Part model, mm, in its own coordinate system. A direction names the side the tool comes from. Give positions to 0.01 mm unless a question says otherwise; leave off trailing zeros. Order: outer loops, then holes, each group sorted by start corner. A loop starts at its lowest first (then second) coordinate and runs counter-clockwise, first axis right, second up. Notation, with made-up numbers: (83.25, -40) -> (95.25, -40) arc R11 cw to (95.25, -24) -> close; hole circle Ø9 at (68, 11.5). An arc over 180 degrees is marked (long way). Write item = value, one per line. Start each with the question number.
Item 1: Flat gauge pins, fed straight in: P1, Ø1.5, axis at x = 5, y = 18.5, coming from the +Z side; P2, Ø1.5, axis at y = 24, z = 7, coming from the -X side; P3, Ø0.6, axis at y = 28.5, z = 6.5, coming from the +X side; P4, Ø2.5, axis at x = 7.5, y = 5, coming from the +Z side. Where does each tip first touch, or does it go through?
Item 2: Band-saw the part on D-D on z = 1.5. Write the cut outline in (x, y).
Item 3: Tool access for faces 1 (the face through (8, 20, 6)), 2 (the face through (8, 28, 7)), 3 (the face through (5, 29, 6)): list every direction of +Z, -Z, +X, -X, +Y, -Y with a clear straight run to the whole face (end or side of a thin tool).
Item 4: Band-saw the part on B-B on x = 7.5. Write the cut outline in (y, z).
Item 5: Drill centre lines: line 1 along Y through (x, z) = (7.5, 3.2); line 2 along Y through (x, z) = (8.75, 5.5); line 3 along X through (y, z) = (15, 3.05). Where is each one in solid material? Low to high.
Item 6: Pull direction Y, two halves, no side cores. Call faces 4 (the face through (7, 0, 2)), 5 (the face through (9, 5, 2)), 6 (the face through (7, 29, 8)): +Y half, -Y half, draft (parallel to the pull), parting line (faces both ways), or undercut.
Item 7: Band-saw the part on C-C on z = 7. Write the cut outline in (x, y).
Item 8: Band-saw the part on A-A on y = 5. Write the cut outline in (x, z), plus the area to 3 significant figures.
Autodesk Fusion 360 part; units mm, degrees
sketch "Sketch1" plane through (0, 0, 0) normal (0, 0, 1) x (1, 0, 0)
  line L0 (0, 0) -> (15, 0)
  line L1 (15, 0) -> (15, 30)
  line L2 (15, 30) -> (0, 30)
  line L3 (0, 30) -> (0, 0)
extrude "Extrude1" add sketch "Sketch1" along normal blind 5
sketch "Sketch2" plane through (0, 0, 5) normal (0, 0, 1) x (1, 0, 0)
  line L0 (0, 30) -> (0, 0)
  line L1 (0, 0) -> (15, 0)
  line L2 (15, 0) -> (15, 30)
  line L3 (15, 30) -> (0, 30)
  line L4 (5, 30) -> (10, 30)
  line L5 (10, 30) -> (10, 20)
  line L6 (10, 20) -> (5, 20)
  line L7 (5, 20) -> (5, 30)
  dimension "d3" = 10
extrude "Extrude2" add sketch "Sketch2" along normal blind 3 contours L3 L4 L5 L6 L7
sketch "Sketch3" plane through (10, 0, 0) normal (1, 0, 0) x (0, 0, -1)
  line L0 (-5, 20) -> (-5, 30)
  line L1 (-5, 30) -> (-8, 30)
  line L2 (-8, 30) -> (-8, 20)
  line L3 (-8, 20) -> (-5, 20)
  line L4 (-8, 28) -> (-5, 28)
  line L5 (-5, 28) -> (-5, 26)
  line L6 (-5, 26) -> (-8, 26)
  line L7 (-8, 26) -> (-8, 28)
  dimension "d6" = 2
  dimension "d7" = 6
extrude "Extrude3" cut sketch "Sketch3" against normal blind 6 contours L0 L2 L4 L5 L6 L7
sketch "Sketch4" plane through (0, 0, 5) normal (0, 0, 1) x (1, 0, 0)
  line L0 (5, 28) -> (5, 30)
  line L1 (5, 30) -> (0, 30)
  line L2 (0, 30) -> (0, 0)
  line L3 (0, 0) -> (15, 0)
  line L4 (15, 0) -> (15, 30)
  line L5 (15, 30) -> (10, 30)
  line L6 (10, 30) -> (10, 28)
  line L7 (10, 28) -> (5, 28)
  line L8 (5, 26) -> (10, 26)
  line L9 (10, 26) -> (10, 20)
  line L10 (10, 20) -> (5, 20)
  line L11 (5, 20) -> (5, 26)
  point P0 (7.5, 5)
  point P1 (7.5, 15)
  dimension "d14" = 5
  dimension "d15" = 15
hole "Hole1" at (7.5, 5, 5) at (7.5, 15, 5) direction (0, 0, -1) diameter 3 end through all
Values found:
q1.P1 = 5
q1.P2 = 5
q1.P3 = 10
q1.P4 = through
q2.outline = (0, 0) -> (15, 0) -> (15, 30) -> (0, 30) -> close; hole circle Ø3 at (7.5, 5); hole circle Ø3 at (7.5, 15)
q3.face_1 = +Z, +X, -X, -Y
q3.face_2 = +Z, +X, -X
q3.face_3 = +Z, -X, +Y, -Y
q4.outline = (0, 0) -> (3.5, 0) -> (3.5, 5) -> (0, 5) -> close; (6.5, 0) -> (13.5, 0) -> (13.5, 5) -> (6.5, 5) -> close; (16.5, 0) -> (30, 0) -> (30, 8) -> (28, 8) -> (28, 5) -> (26, 5) -> (26, 8) -> (20, 8) -> (20, 5) -> (16.5, 5) -> close
q5.line_1 = 0 to 3.5, 6.5 to 13.5, 16.5 to 30
q5.line_2 = 20 to 26, 28 to 30
q5.line_3 = 0 to 6, 9 to 15
q6.face_4 = -Y half
q6.face_5 = undercut
q6.face_6 = draft
q7.outline = (5, 20) -> (10, 20) -> (10, 26) -> (5, 26) -> close; (5, 28) -> (10, 28) -> (10, 30) -> (5, 30) -> close
q8.outline = (0, 0) -> (6, 0) -> (6, 5) -> (0, 5) -> close; (9, 0) -> (15, 0) -> (15, 5) -> (9, 5) -> close
q8.area = 60.0 mm^2
